Can you work these out from the model? Positions are in its coordinate system, mm. Round coordinates to 2 decimals unless told otherwise and drop trailing zeros. Loops run counter-clockwise (first coordinate to the right, second up) from the corner with the lowest first, then second, coordinate; pieces in that order, holes last.
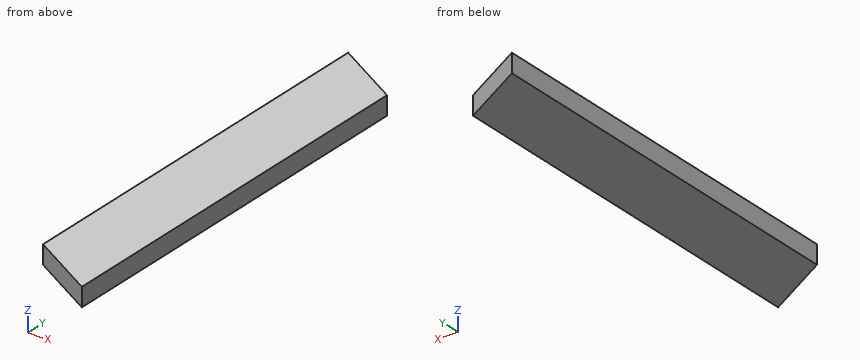
from build123d import *

# Parameters (mm, degrees)
F0_W     = 139.7
F0_H     = 38.1
F1_DEPTH = 914.4
F3_DEPTH = 50.8
F5_DEPTH = 50.8


with BuildPart() as f1:
    # F0 (on Front) → F1 (new body)
    with BuildSketch(Plane.XZ):
        with Locations((69.85, 19.05)):
            Rectangle(F0_W, F0_H)
    extrude(amount=F1_DEPTH)

    # F2 (on Top) → F3 (cut)
    with BuildSketch(Plane.XY):
        Polygon((152.4, 0), (0, 0), (152.4, -87.988181), align=None)
    extrude(amount=F3_DEPTH, mode=Mode.SUBTRACT)

    # F4 (on Top) → F5 (cut)
    with BuildSketch(Plane.XY):
        Polygon((139.7, -914.4), (-12.7, -826.411819), (-12.7, -914.4), align=None)
    extrude(amount=F5_DEPTH, mode=Mode.SUBTRACT)


solid = f1.part
(1) If we section it at B-B, the plane z = 6.5: List the corners of the cut face in (x, y) for me, then the cut area to 3 significant figures.
Worked answers:
outline: (0, -833.74) - (139.7, -914.4) - (139.7, -80.66) - (0, 0) - close
area: 116,000 mm2
(2) Will these pins go through, and if not, where does the flat tip stop? P1, Ø4, axis at y = -710.5, z = 31.5, coming from the -X side; P2, Ø2, axis at x = 29.5, z = 10.5, coming from the -Y side.
Worked answers:
P1: stops at x = 0
P2: stops at y = -851.35
(3) If we section it at A-A, the plane y = -59.5: List the corners of the cut face in (x, z) for me.
Worked answers:
outline: (0, 0) - (103.06, 0) - (103.06, 38.1) - (0, 38.1) - close
(4) If I drill on line 1 (Y direction, x = 51.5, z = 8.5); line 2 (Y direction, x = 34, z = 17.5), over which ranges is the centre line in solid material (lowest first)?
Worked answers:
line 1: y = -863.48 to -29.73
line 2: y = -853.37 to -19.63
